Source: three-view drawing plus pictorial views. Frame: mm from the lowest corner of the part. Give positions to 0.01 mm unless a question says otherwise; leave off trailing zeros. Write each loop counter-clockwise with the first axis right and the second up, starting at its lowest first coordinate (ties: lowest second). Pieces come first, ordered by that corner, then holes. Notation, with made-up numbers: (-35.75, -22.75) -> (12.25, -22.75) arc R12 ccw to (12.25, -14.75) -> close; hole circle Ø9 at (-17, 82). An arc over 180 degrees is marked (long way). Write item = value, one per line.
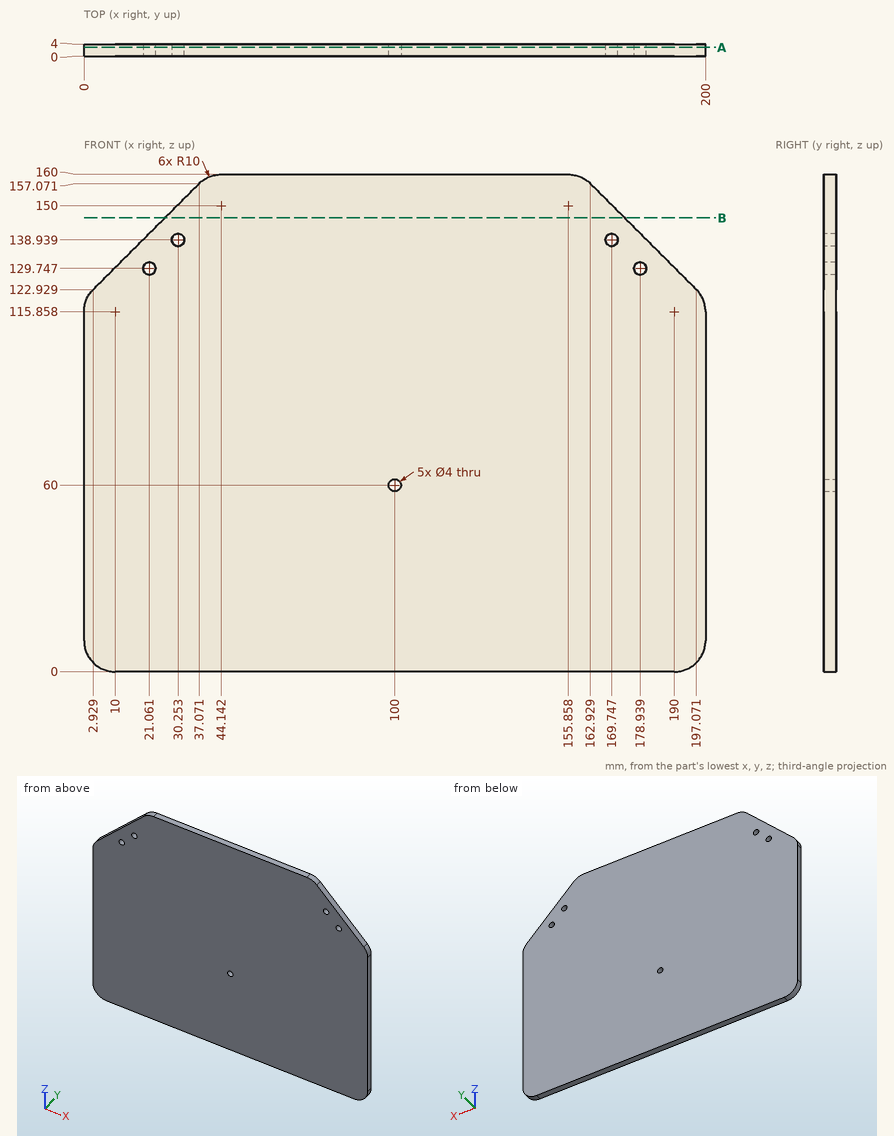
1) Material intervals for L1, parallel to X at y = 2.1, z = 130 (1 decimal); L2, parallel to Z at x = 100, y = 2.05; L3, parallel to X at y = 2.65, z = 136.5, sorted ascending.
Computed:
L1 = 10 to 19.1, 23 to 177, 180.9 to 190
L2 = 0 to 58, 62 to 160
L3 = 16.5 to 183.5
2) Cut plane B-B (z = 146). Return the cut outline in (x, y), then the cut area to 3 significant figures.
Computed:
outline = (26, 0) -> (174, 0) -> (174, 4) -> (26, 4) -> close
area = 592 mm²
3) Cut plane A-A (y = 2.95). Return the cut outline in (x, z).
Computed:
outline = (0, 10) arc R10 ccw to (10, 0) -> (190, 0) arc R10 ccw to (200, 10) -> (200, 115.86) arc R10 ccw to (197.07, 122.93) -> (162.93, 157.07) arc R10 ccw to (155.86, 160) -> (44.14, 160) arc R10 ccw to (37.07, 157.07) -> (2.93, 122.93) arc R10 ccw to (0, 115.86) -> close; hole circle Ø4 at (21.06, 129.75); hole circle Ø4 at (30.25, 138.94); hole circle Ø4 at (100, 60); hole circle Ø4 at (169.75, 138.94); hole circle Ø4 at (178.94, 129.75)
